Could you check a few things on this drawing? It's one solid part, dimensions in mm from its lowest x, y, z. A direction names the side the tool comes from. Give positions to 0.01 mm unless a question says otherwise; leave off trailing zeros. Order: outer loops, then holes, each group sorted by start corner. A loop starts at its lowest first (then second) coordinate and runs counter-clockwise, first axis right, second up.
(1) Imagine slicing it at D-D, the plane z = 21. Write out the boundary of the cut face in (x, y), then the cut area to 3 significant figures.
(2) Will these pins go through, and if not, where does the flat tip stop? pin 1 (10 mm diameter, centred on x = 21, y = 10.5, fed in from -Z); pin 2 (12 mm diameter, centred on y = 11, z = 3.5, fed in from +X); pin 3 (1.5 mm diameter, centred on y = 25, z = 13.5, fed in from +X).
(3) Imagine slicing it at C-C, the plane y = 2. Write out the boundary of the cut face in (x, z), then the cut area to 3 significant figures.
(4) Imagine slicing it at B-B, the plane x = 13.45. Write out the boundary of the cut face in (y, z), then the cut area to 3 significant figures.
(5) If I drill on probe 1 along X at (y, z) = (0.7, 13.45); probe 2 along Y at (x, z) = (6.5, 19); probe 3 along Y at (x, z) = (26, 17), over which ranges is the centre line in solid material (lowest first)?
(6) Imagine slicing it at A-A, the plane z = 13.45. Write out the boundary of the cut face in (x, y), then the cut area to 3 significant figures.
(7) If we mould it in two halves opening along Y, with no side actions, what happens to the marked faces 1, 2, 3 and 4? For each: released by +Y, released by -Y, zero draft, split by the parting line, or undercut.
(8) On a 3-axis mill with a long thin cutter (end or side, diameter ignored), from which of +Z, -Z, +X, -X, +Y, -Y can I reach the whole of each face in a straight line? I mean the marked faces 5, 6 and 7. Say none if no direction works.
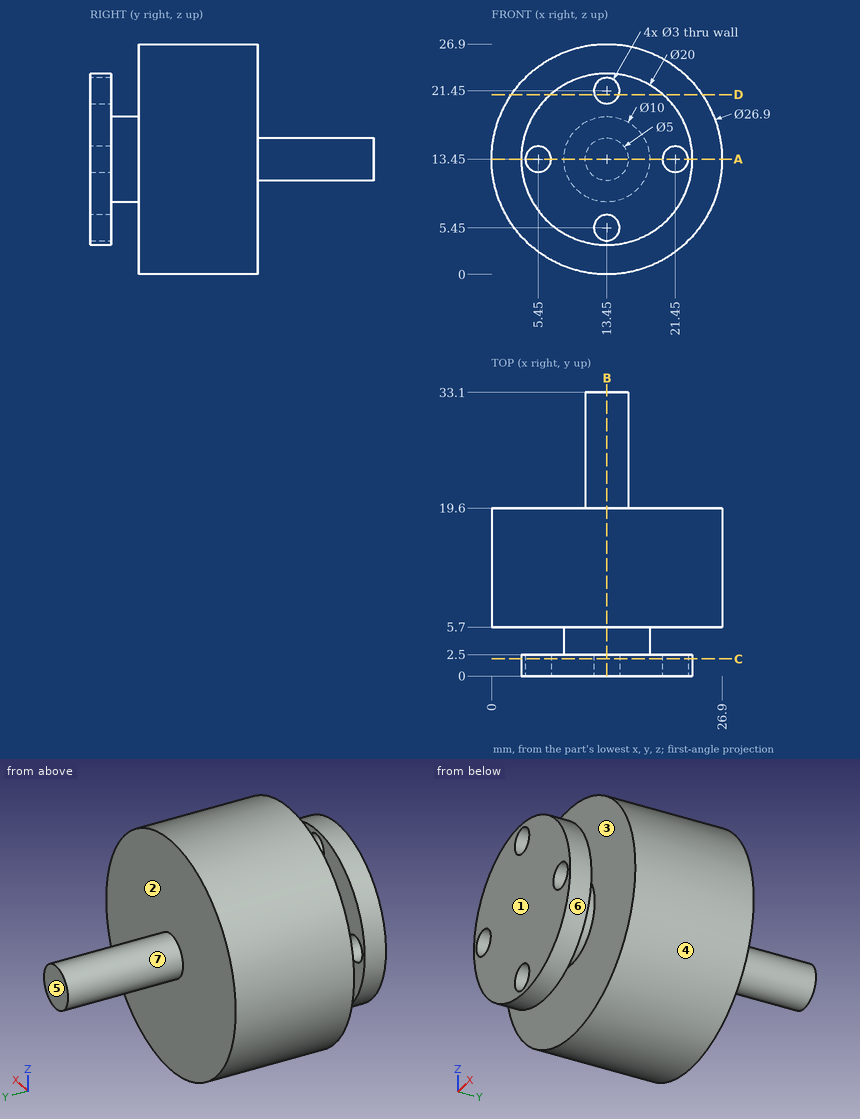
Answer block:
1. outline: (2.32, 5.7) - (24.58, 5.7) - (24.58, 19.6) - (2.32, 19.6) - close; (6.89, 0) - (12.02, 0) - (12.02, 2.5) - (6.89, 2.5) - close; (14.88, 0) - (20.01, 0) - (20.01, 2.5) - (14.88, 2.5) - close
1. area: 335 mm2
2. pin 1: stops at z = 0.24
2. pin 2: stops at x = 26.31
2. pin 3: stops at x = 15.95
3. outline: circle Ø20 at (13.45, 13.45); hole circle Ø3 at (5.45, 13.45); hole circle Ø3 at (13.45, 5.45); hole circle Ø3 at (13.45, 21.45); hole circle Ø3 at (21.45, 13.45)
3. area: 286 mm2
4. outline: (0, 3.45) - (2.5, 3.45) - (2.5, 3.95) - (0, 3.95) - close; (0, 6.95) - (2.5, 6.95) - (2.5, 8.45) - (5.7, 8.45) - (5.7, 0) - (19.6, 0) - (19.6, 10.95) - (33.1, 10.95) - (33.1, 15.95) - (19.6, 15.95) - (19.6, 26.9) - (5.7, 26.9) - (5.7, 18.45) - (2.5, 18.45) - (2.5, 19.95) - (0, 19.95) - close; (0, 22.95) - (2.5, 22.95) - (2.5, 23.45) - (0, 23.45) - close
4. area: 508 mm2
5. probe 1: x = 3.45 to 3.95, 6.95 to 19.95, 22.95 to 23.45
5. probe 2: y = 0 to 2.5, 5.7 to 19.6
5. probe 3: y = 5.7 to 19.6
6. outline: (0, 5.7) - (8.45, 5.7) - (8.45, 2.5) - (6.95, 2.5) - (6.95, 0) - (19.95, 0) - (19.95, 2.5) - (18.45, 2.5) - (18.45, 5.7) - (26.9, 5.7) - (26.9, 19.6) - (15.95, 19.6) - (15.95, 33.1) - (10.95, 33.1) - (10.95, 19.6) - (0, 19.6) - close; (3.45, 0) - (3.95, 0) - (3.95, 2.5) - (3.45, 2.5) - close; (22.95, 0) - (23.45, 0) - (23.45, 2.5) - (22.95, 2.5) - close
6. area: 508 mm2
7. face 1: released by -Y
7. face 2: released by +Y
7. face 3: undercut
7. face 4: zero draft
8. face 5: +Z, -Z, +X, -X, +Y
8. face 6: -Y
8. face 7: +Y
